Build history of the part. All positions in model axes, mm. Face numbers are marked on the shaded views. A direction names the side the tool comes from. Round coordinates to 2 decimals unless told otherwise and drop trailing zeros. Order: outer loops, then holes, each group sorted by start corner. A loop starts at its lowest first (then second) coordinate and runs counter-clockwise, first axis right, second up. Notation, with made-up numbers: (-15.75, -37) -> (7.25, -37) arc R11 ccw to (7.25, -31) -> close; hole circle Ø11 at (-3, 82). An arc over 180 degrees is marked (long way). Answer as CSV lines item,"result". Start each with the question number.
```python
from build123d import *

# Parameters (mm, degrees)
F0_W     = 125.408068
F0_H     = 30
F0_W_2   = 100
F0_H_2   = 1500
F1_DEPTH = 640
F3_DEPTH = 1730.001
F5_DEPTH = 2114.592932


with BuildPart() as f1:
    # F0 (on Top) → F1 (new body)
    with BuildSketch(Plane.XY):
        Polygon((0, 100), (0, 0), (1140, 0), (1140, 100), (1014.591932, 100), align=None)
        with Locations((1077.295966, 115)):
            Rectangle(F0_W, F0_H)
        Polygon((1014.591932, 130), (1140, 130), (2114.591932, 130), (2114.591932, 230), (2014.591932, 230), (1014.591932, 230), align=None)
        with Locations((2064.591932, 980)):
            Rectangle(F0_W_2, F0_H_2)
    extrude(amount=F1_DEPTH)

    # F2 (on face) → F3 (cut, through all)
    with BuildSketch(Plane.XZ):
        Polygon((162.857143, 450), (0, 450), (0, 0), (977.142857, 0), (977.142857, 75), (814.285714, 75), (814.285714, 150), (651.428571, 150), (651.428571, 225), (488.571429, 225), (488.571429, 300), (325.714286, 300), (325.714286, 375), (162.857143, 375), align=None)
    extrude(amount=-F3_DEPTH, mode=Mode.SUBTRACT)

    # F4 (on face) → F5 (cut, through all)
    with BuildSketch(Plane.YZ.offset(2114.591932)):
        Polygon((1272.857143, 375), (1272.857143, 300), (1044.285714, 300), (1044.285714, 225), (815.714286, 225), (815.714286, 150), (587.142857, 150), (587.142857, 75), (358.571429, 75), (358.571429, 0), (1730, 0), (1730, 450), (1501.428571, 450), (1501.428571, 375), align=None)
    extrude(amount=-F5_DEPTH, mode=Mode.SUBTRACT)


solid = f1.part
```
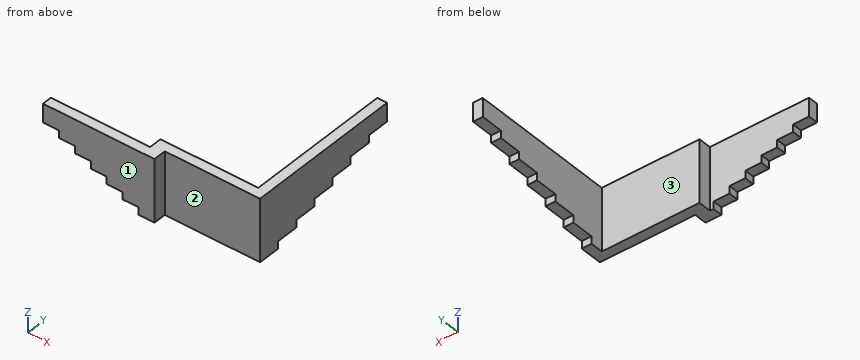
Q1. Slice it at C-C, the plane x = 200. Write the cut outline in (y, z).
Q2. Slice it at B-B, the plane y = 554.5. Write the cut outline in (x, z).
Q3. Flat gauge pins, fed straight in: pin 1 Ø5 at (x, z) = (1413, 386.5) entering from +Y; pin 2 Ø22.5 at (y, z) = (51.5, 104.5) entering from -X; pin 3 Ø10 at (x, z) = (1520.5, 409) entering from -Y. Where does each tip first touch, or does it go through?
Q4. Slice it at A-A, the plane z = 541. Write the cut outline in (x, y).
Q5. Probe L1, parallel to X at y = 1541.5, z = 527.5; L2, parallel to Y at x = 554, z = 444.5; L3, parallel to Y at x = 1582.5, z = 251.5. List the from-to ranges inside material, lowest first.
Q6. Which spindle directions (+Z, -Z, +X, -X, +Y, -Y) get a long thin tool onto all of the face, cutting with end or side? Do the marked faces 1, 2 and 3. Say none if no direction does.
Q7. Slice it at D-D, the plane z = 49. Write the cut outline in (x, y).
Solutions:
1,outline,"(0, 375) -> (100, 375) -> (100, 640) -> (0, 640) -> close"
2,outline,"(2014.59, 75) -> (2114.59, 75) -> (2114.59, 640) -> (2014.59, 640) -> close"
3,pin 1,"stops at y = 230"
3,pin 2,"stops at x = 814.29"
3,pin 3,"stops at y = 130"
4,outline,"(0, 0) -> (1140, 0) -> (1140, 130) -> (2114.59, 130) -> (2114.59, 1730) -> (2014.59, 1730) -> (2014.59, 230) -> (1014.59, 230) -> (1014.59, 100) -> (0, 100) -> close"
5,L1,"x = 2014.59 to 2114.59"
5,L2,"y = 0 to 100"
5,L3,"y = 130 to 230"
6,face 1,"+Z, -Z, +X, -X, -Y"
6,face 2,"+Z, -Z, +X, -Y"
6,face 3,"+Z, -Z, -X, +Y"
7,outline,"(977.14, 0) -> (1140, 0) -> (1140, 130) -> (2114.59, 130) -> (2114.59, 358.57) -> (2014.59, 358.57) -> (2014.59, 230) -> (1014.59, 230) -> (1014.59, 100) -> (977.14, 100) -> close"
